Could you check a few things on this drawing? It's one solid part, dimensions in mm from its lowest x, y, z. Round coordinates to 2 decimals unless told otherwise and drop trailing zeros. Loops run counter-clockwise (first coordinate to the right, second up) from the corner with the lowest first, then second, coordinate; pieces in that order, holes last. Notation, with made-up numbers: M -22,68.5 L 34,68.5 A15 ccw 34,79.5 Z; hole C 64,-28.5 d7. An arc over 180 degrees is marked long. Write item = value, one per line. Start each with the question number.
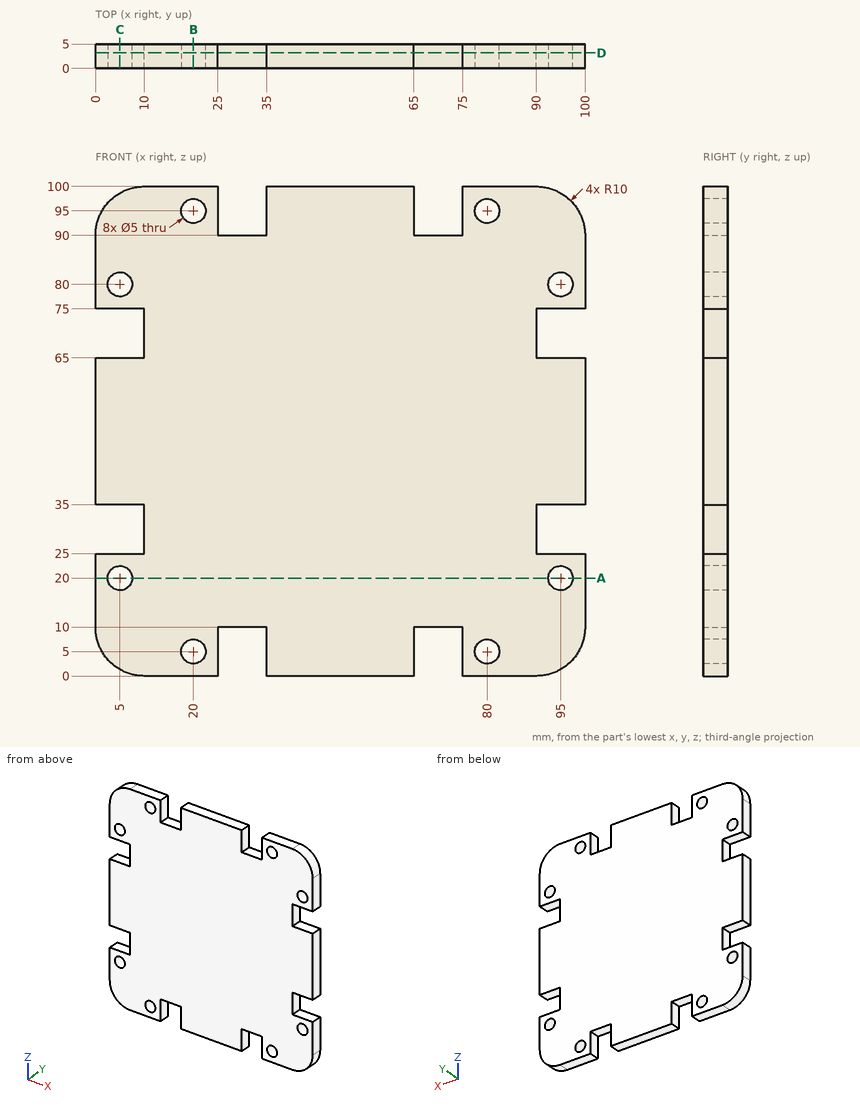
Item 1: I want a section at D-D, the plane y = 3.2. State how many separate pieces and enclosed holes the cut face has, then the cut area to 3 significant figures.
Item 2: Please list where these lines run through material, in increasing order: line 1 (Z direction, x = 80, y = 1.85); line 2 (Z direction, x = 21, y = 4.05). Write a range as [from, to].
Item 3: I want a section at B-B, the plane x = 20. List the corners of the cut face in (y, z) for me.
Item 4: I want a section at A-A, the plane z = 20. List the corners of the cut face in (x, y) for me, then the cut area to 3 significant figures.
Item 5: I want a section at C-C, the plane x = 5. List the corners of the cut face in (y, z) for me, then the cut area to 3 significant figures.
Item 6: Will these pins go through, and if not, where does the flat tip stop? pin 1 Ø1.5 at (x, y) = (3, 3) entering from -Z; pin 2 Ø1.5 at (x, y) = (28.5, 3) entering from -Z; pin 3 Ø3 at (x, z) = (95, 20) entering from -Y; pin 4 Ø2 at (y, z) = (0.5, 33) entering from +X.
Worked out:
q1.separate_pieces = 1
q1.enclosed_holes = 8
q1.area = 8,960 mm2
q2.line_1 = [0, 2.5], [7.5, 92.5], [97.5, 100]
q2.line_2 = [0, 2.71], [7.29, 92.71], [97.29, 100]
q3.outline = M 0,0 L 5,0 L 5,2.5 L 0,2.5 Z; M 0,7.5 L 5,7.5 L 5,92.5 L 0,92.5 Z; M 0,97.5 L 5,97.5 L 5,100 L 0,100 Z
q4.outline = M 0,0 L 2.5,0 L 2.5,5 L 0,5 Z; M 7.5,0 L 92.5,0 L 92.5,5 L 7.5,5 Z; M 97.5,0 L 100,0 L 100,5 L 97.5,5 Z
q4.area = 450 mm2
q5.outline = M 0,1.34 L 5,1.34 L 5,17.5 L 0,17.5 Z; M 0,22.5 L 5,22.5 L 5,25 L 0,25 Z; M 0,35 L 5,35 L 5,65 L 0,65 Z; M 0,75 L 5,75 L 5,77.5 L 0,77.5 Z; M 0,82.5 L 5,82.5 L 5,98.66 L 0,98.66 Z
q5.area = 337 mm2
q6.pin_1 = 2.19
q6.pin_2 = 10
q6.pin_3 = through
q6.pin_4 = 90
